For this review, take the finished solid that the model builds, in its own axes (mm). A direction names the side the tool comes from. Coordinates: 2 decimals unless noted, no trailing zeros. Loops run counter-clockwise (first coordinate to the right, second up) from the corner with the lowest first, then second, coordinate; pieces in that order, holes last.
1. Mouldability with a two-part tool opening along Z and no side actions: class faces 3 (the face through (0.15, -3, 4)), 4 (the face through (4.15, 4, 7)), 5 (the face through (-1, 4, 0)) as pulls with the +Z half, pulls with the -Z half, needs draft (parallel to the pull), parting line crosses it, or undercut.
2. Take a section at C-C, the plane y = -1.25. State the section outline as (x, z) points.
3. Machinability: for faces 1 (the face through (-1, 14.175, 7)), 2 (the face through (2.178, -1.692, 0.595)), which of the approach directions +Z, -Z, +X, -X, +Y, -Y give a long, thin tool a straight path to every point of the face, cutting with its end or side? Answer none if there is none.
4. Take a section at D-D, the plane z = 4.75. State the section outline as (x, y) points.
5. Take a section at B-B, the plane x = -1.5. State the section outline as (y, z) points.
6. Clearance check with flat-ended pins moving along their axes: P1, Ø6.5, axis at y = -2.5, z = 6, coming from the +X side; P2, Ø6.5, axis at y = -0.82, z = 4.5, coming from the +X side. State where each tip first meets the part, or that it passes through.
7. To check wall thickness, follow probe 1 along Y at (x, z) = (0, 2.75); probe 2 along X at (y, z) = (2, 4.5); probe 3 along Y at (x, z) = (-2.5, 11.25). State the ranges of each line that lie inside material, in increasing order.
8. Take a section at A-A, the plane z = 6.25. State the section outline as (x, y) points, then the cut area to 3 significant figures.
```python
from build123d import *

# Parameters (mm, degrees)
F0_W     = 10
F0_H     = 20
F1_DEPTH = 15
F2_R     = 2
F3_DEPTH = 20
F2_R_2   = 4
F4_DEPTH = 4
F5_R     = 2
F6_DEPTH = 20


with BuildPart() as f1:
    # F0 (on Top) → F1 (new body)
    with BuildSketch(Plane.XY):
        with Locations((-0.84982, 4.175278)):
            Rectangle(F0_W, F0_H)
    extrude(amount=F1_DEPTH)

    # F2 (on face) → F3 (cut)
    with BuildSketch(Plane.YZ.offset(4.15018)):
        with Locations((-0.824722, 4.5)):
            Circle(F2_R)
    extrude(amount=-F3_DEPTH, mode=Mode.SUBTRACT)

    # F2 (on face) → F4 (cut)
    with BuildSketch(Plane.YZ.offset(4.15018)):
        with Locations((-0.824722, 4.5)):
            Circle(F2_R_2)
        with Locations((-0.824722, 4.5)):
            Circle(F2_R, mode=Mode.SUBTRACT)
    extrude(amount=-F4_DEPTH, mode=Mode.SUBTRACT)

    # F5 (on face) → F6 (cut)
    with BuildSketch(Plane.XY.offset(15)):
        with Locations((-0.84982, 9.175278)):
            Circle(F5_R)
    extrude(amount=-F6_DEPTH, mode=Mode.SUBTRACT)


solid = f1.part
```
Results list:
1. face 3: undercut
1. face 4: needs draft
1. face 5: pulls with the -Z half
2. outline: (-5.85, 0) - (4.15, 0) - (4.15, 0.52) - (0.15, 0.52) - (0.15, 2.55) - (-5.85, 2.55) - close; (-5.85, 6.45) - (0.15, 6.45) - (0.15, 8.48) - (4.15, 8.48) - (4.15, 15) - (-5.85, 15) - close
3. face 1: +Z, -Z, +X, -X, +Y
3. face 2: +X
4. outline: (-5.85, -5.82) - (4.15, -5.82) - (4.15, -4.82) - (0.15, -4.82) - (0.15, -2.81) - (-5.85, -2.81) - close; (-5.85, 1.16) - (0.15, 1.16) - (0.15, 3.17) - (4.15, 3.17) - (4.15, 14.18) - (-5.85, 14.18) - close; hole circle Ø4 at (-0.85, 9.18)
5. outline: (-5.82, 0) - (7.28, 0) - (7.28, 15) - (-5.82, 15) - close; (11.07, 0) - (14.18, 0) - (14.18, 15) - (11.07, 15) - close; hole circle Ø4 at (-0.82, 4.5)
6. P1: stops at x = 4.15
6. P2: stops at x = 0.15
7. probe 1: y = -5.82 to -1.79, 0.14 to 7.36, 10.99 to 14.18
7. probe 2: x = -5.85 to 0.15
7. probe 3: y = -5.82 to 8.05, 10.31 to 14.18
8. outline: (-5.85, -5.82) - (4.15, -5.82) - (4.15, -4.42) - (0.15, -4.42) - (0.15, -1.79) - (-5.85, -1.79) - close; (-5.85, 0.14) - (0.15, 0.14) - (0.15, 2.77) - (4.15, 2.77) - (4.15, 14.18) - (-5.85, 14.18) - close; hole circle Ø4 at (-0.85, 9.18)
8. area: 147 mm2
